Answer from the drawing. Dimensions are ordinates in mm from the lowest x, y and z of the part. A direction names the side the tool comes from. Coordinates: 2 decimals unless noted, no trailing zeros. Loops run counter-clockwise (first coordinate to the right, second up) from the corner with the lowest first, then second, coordinate; pieces in that order, holes last.
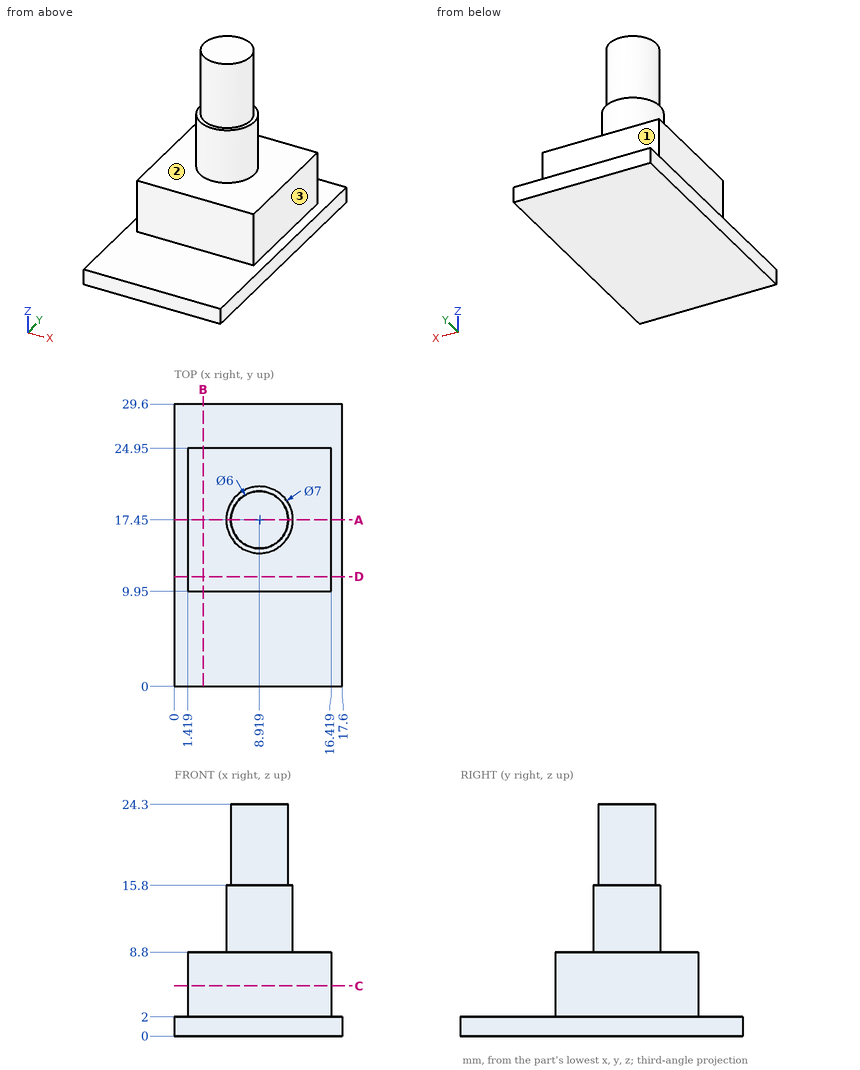
Item 1: A cutting plane is placed at A-A on y = 17.45. Determine the outline of the cut face in (x, z), then the cut area to 3 significant figures.
Numbers:
outline: (0, 0) - (17.6, 0) - (17.6, 2) - (16.42, 2) - (16.42, 8.8) - (12.42, 8.8) - (12.42, 15.8) - (11.92, 15.8) - (11.92, 24.3) - (5.92, 24.3) - (5.92, 15.8) - (5.42, 15.8) - (5.42, 8.8) - (1.42, 8.8) - (1.42, 2) - (0, 2) - close
area: 237 mm2
Item 2: Which of the six approach directions +Z, -Z, +X, -X, +Y, -Y give full straight-line access (tool end or side, diameter ignored) to the marked faces 1, 2 and 3?
Numbers:
face 1: +Z, +X, -X, +Y
face 2: +Z
face 3: +Z, +X, +Y, -Y
Item 3: A cutting plane is placed at B-B on x = 3. Determine the outline of the cut face in (y, z), then the cut area to 3 significant figures.
Numbers:
outline: (0, 0) - (29.6, 0) - (29.6, 2) - (24.95, 2) - (24.95, 8.8) - (9.95, 8.8) - (9.95, 2) - (0, 2) - close
area: 161 mm2
Item 4: Given pin 1 (8 mm diameter, centred on x = 9.5, z = 18.5, fed in from -Y); pin 2 (2 mm diameter, centred on y = 17, z = 7, fed in from -X); pin 3 (3 mm diameter, centred on x = 4.5, z = 11.5, fed in from -Y); pin 4 (6 mm diameter, centred on y = 25, z = 18.5, fed in from -X) (3 decimals), each flat-ended and moving along its own axis, determine where each tip first touches the part or whether it passes through.
Numbers:
pin 1: stops at y = 13.95
pin 2: stops at x = 1.42
pin 3: stops at y = 15.52
pin 4: passes through
Item 5: Find the intervals of material crossed by line 1 along Y through (x, z) = (16.25, 6); line 2 along Z through (x, y) = (10, 26); line 3 along Z through (x, y) = (10.75, 21.25), in increasing order.
Numbers:
line 1: y = 9.95 to 24.95
line 2: z = 0 to 2
line 3: z = 0 to 8.8
Item 6: A cutting plane is placed at C-C on z = 5.25. Determine the outline of the cut face in (x, y), then the cut area to 3 significant figures.
Numbers:
outline: (1.42, 9.95) - (16.42, 9.95) - (16.42, 24.95) - (1.42, 24.95) - close
area: 225 mm2
Item 7: A cutting plane is placed at D-D on y = 11.5. Determine the outline of the cut face in (x, z).
Numbers:
outline: (0, 0) - (17.6, 0) - (17.6, 2) - (16.42, 2) - (16.42, 8.8) - (1.42, 8.8) - (1.42, 2) - (0, 2) - close
